Model file for the job. Use its own axes, mm. A direction names the side the tool comes from. Round coordinates to 2 decimals unless told otherwise and drop trailing zeros. Order: outer loops, then holes, each group sorted by start corner. A loop starts at its lowest first (then second) coordinate and runs counter-clockwise, first axis right, second up. Notation, with made-up numbers: (73, 9.25) - (125, 9.25) arc R8 cw to (125, 21.25) - close; hole circle Ø5 at (83, -20). An arc over 180 degrees is marked (long way). Write item = value, one per line.
```python
from build123d import *

# Parameters (mm, degrees)
F0_W     = 170
F0_H     = 50
F0_R     = 2.25
F0_R_2   = 1.75
F1_DEPTH = 2
F2_R     = 3
F3_R     = 1.5


# Not quite as in the source:
# - a feature names something its author has since deleted; it is built from what else it names


with BuildPart() as f1:
    # F0 (on Front) → F1 (new body)
    with BuildSketch(Plane.XZ):
        with Locations((85, 25)):
            Rectangle(F0_W, F0_H)
        with Locations((7.5, 25)):
            Circle(F0_R, mode=Mode.SUBTRACT)
        with BuildLine():
            Line((27.5, 27), (33, 27))
            Line((33, 27), (33, 32.5))
            ThreePointArc((33, 32.5), (35, 34.5), (37, 32.5))
            Line((37, 32.5), (37, 27))
            Line((37, 27), (42.5, 27))
            ThreePointArc((42.5, 27), (44.5, 25), (42.5, 23))
            Line((42.5, 23), (37, 23))
            Line((37, 23), (37, 17.5))
            ThreePointArc((37, 17.5), (35, 15.5), (33, 17.5))
            Line((33, 17.5), (33, 23))
            Line((33, 23), (27.5, 23))
            ThreePointArc((27.5, 23), (25.5, 25), (27.5, 27))
        make_face(mode=Mode.SUBTRACT)
        with Locations((85, 25)):
            Circle(F0_R_2, mode=Mode.SUBTRACT)
        with BuildLine():
            ThreePointArc((127.5, 23), (125.5, 25), (127.5, 27))
            Line((127.5, 27), (133, 27))
            Line((133, 27), (133, 32.5))
            ThreePointArc((133, 32.5), (135, 34.5), (137, 32.5))
            Line((137, 32.5), (137, 27))
            Line((137, 27), (142.5, 27))
            ThreePointArc((142.5, 27), (144.5, 25), (142.5, 23))
            Line((142.5, 23), (137, 23))
            Line((137, 23), (137, 17.5))
            ThreePointArc((137, 17.5), (135, 15.5), (133, 17.5))
            Line((133, 17.5), (133, 23))
            Line((133, 23), (127.5, 23))
        make_face(mode=Mode.SUBTRACT)
        with Locations((162.5, 25)):
            Circle(F0_R, mode=Mode.SUBTRACT)
    extrude(amount=F1_DEPTH)

    # F2
    f2_edges = [f1.edges().sort_by_distance(p)[0] for p in [
        (33, -1, 27),
        (37, -1, 27),
        (37, -1, 23),
        (33, -1, 23),
        (133, -1, 27),
        (133, -1, 23),
        (137, -1, 27),
        (137, -1, 23),
    ]]
    fillet(f2_edges, radius=F2_R)

    # F3
    f3_edges = [f1.edges().sort_by_distance(p)[0] for p in [
        (0, -1, 50),
        (0, -1, 0),
        (170, -1, 50),
        (170, -1, 0),
    ]]
    fillet(f3_edges, radius=F3_R)


solid = f1.part
```
1) Flat gauge pin, fed straight in: pin 1 Ø2 at (x, z) = (20.5, 15) entering from +Y. Where does the tip first touch, or does it go through?
Conclusion:
pin_1 = 0
2) Cut at A-A (z = 25). Write the cut outline in (x, y).
Conclusion:
outline = (0, -2) - (5.25, -2) - (5.25, 0) - (0, 0) - close; (9.75, -2) - (25.5, -2) - (25.5, 0) - (9.75, 0) - close; (44.5, -2) - (83.25, -2) - (83.25, 0) - (44.5, 0) - close; (86.75, -2) - (125.5, -2) - (125.5, 0) - (86.75, 0) - close; (144.5, -2) - (160.25, -2) - (160.25, 0) - (144.5, 0) - close; (164.75, -2) - (170, -2) - (170, 0) - (164.75, 0) - close
3) Cut at C-C (y = -0.6). Give the number of separate pieces and of enclosed holes in the cut face, and give its area (3 significant figures).
Conclusion:
separate_pieces = 1
enclosed_holes = 5
area = 8,180 mm^2
4) Wall check: line 1 along Z through (x, y) = (162.5, -0.6); line 2 along X through (y, z) = (-0.95, 17.5); line 3 along Z through (x, y) = (85, -0.9). Give the ranges that are in metal, low to high.
Conclusion:
line_1 = 0 to 22.75, 27.25 to 50
line_2 = 0 to 33, 37 to 133, 137 to 170
line_3 = 0 to 23.25, 26.75 to 50
5) Cut at B-B (x = 85). Write the cut outline in (y, z).
Conclusion:
outline = (-2, 0) - (0, 0) - (0, 23.25) - (-2, 23.25) - close; (-2, 26.75) - (0, 26.75) - (0, 50) - (-2, 50) - close
6) Cut at D-D (x = 135). Write the cut outline in (y, z), and give its area (3 significant figures).
Conclusion:
outline = (-2, 0) - (0, 0) - (0, 15.5) - (-2, 15.5) - close; (-2, 34.5) - (0, 34.5) - (0, 50) - (-2, 50) - close
area = 62.0 mm^2
7) 3-axis set-ups, long thin cutter, end or side, ignore diameter. For faces 1 (the face through (84, -2, 31)), 2 (the face through (132.1, -1.01, 22.14)): which of +Z, -Z, +X, -X, +Y, -Y reach the whole face in a straight line?
Conclusion:
face_1 = +Z, -Z, +X, -X, -Y
face_2 = +Y, -Y
8) Mould opens along Z. For faces 3 (the face through (164.58, -0.99, 24.14)), 4 (the face through (84, 0, 31)) say: +Z half, -Z half, draft (parallel to the pull), parting line (faces both ways), or undercut.
Conclusion:
face_3 = undercut
face_4 = draft
